The drawing under review shows one solid part. Ordinate dimensions are in mm from its lowest x, y, z. Coordinates: 2 decimals unless noted, no trailing zeros. Write each loop counter-clockwise with the first axis right and the second up, starting at its lowest first coordinate (ties: lowest second). Pieces come first, ordered by that corner, then holes. Notation, with made-up numbers: M -8.5,73 L 49.5,73 A20 cw 49.5,105 Z; hole C 16.25,-28.5 d2. An arc over 180 degrees is marked long. Write item = value, one per line.
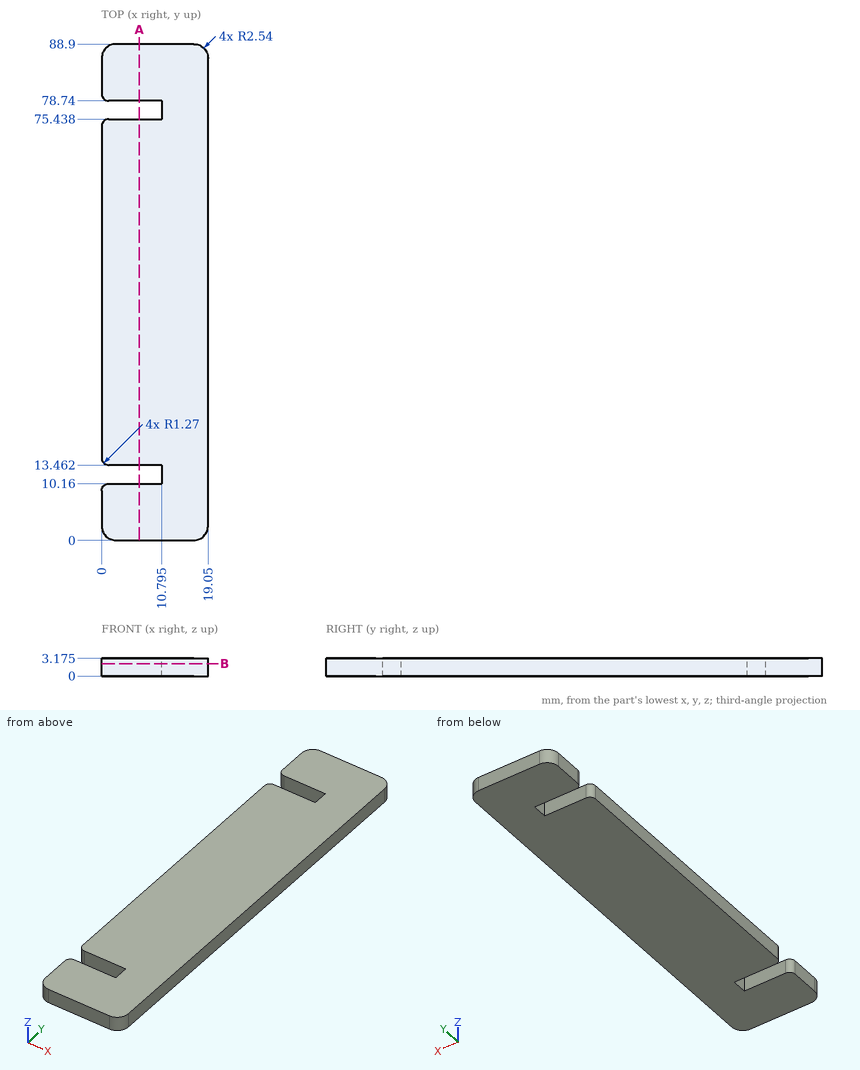
Q1. For P1, Ø1.6, axis at y = 11, z = 1.5, coming from the -X side (3 decimals), flat-tipped, find the tip position at first contact; note if it passes through.
Check result:
P1 = 10.795
Q2. Consider section B-B, the plane z = 2.2. State the section outline as (x, y) points (3 decimals), and give its area (3 significant figures).
Check result:
outline = M 0,2.54 A2.54 ccw 2.54,0 L 16.51,0 A2.54 ccw 19.05,2.54 L 19.05,86.36 A2.54 ccw 16.51,88.9 L 2.54,88.9 A2.54 ccw 0,86.36 L 0,80.01 A1.27 ccw 1.27,78.74 L 10.795,78.74 L 10.795,75.438 L 1.27,75.438 A1.27 ccw 0,74.168 L 0,14.732 A1.27 ccw 1.27,13.462 L 10.795,13.462 L 10.795,10.16 L 1.27,10.16 A1.27 ccw 0,8.89 Z
area = 1,620 mm²
Q3. Wall thickness on line 1 (Y direction, x = 6, z = 0.3); line 2 (X direction, y = 14.5, z = 1): over which ranges is each line inside the solid? List them lowest first.
Check result:
line_1 = 0 to 10.16, 13.46 to 75.44, 78.74 to 88.9
line_2 = 0.02 to 19.05
Q4. Consider section A-A, the plane x = 6.75. State the section outline as (y, z) points (3 decimals), and give its area (3 significant figures).
Check result:
outline = M 0,0 L 10.16,0 L 10.16,3.175 L 0,3.175 Z; M 13.462,0 L 75.438,0 L 75.438,3.175 L 13.462,3.175 Z; M 78.74,0 L 88.9,0 L 88.9,3.175 L 78.74,3.175 Z
area = 261 mm²
